Autodesk Inventor part; units mm, degrees
ref_plane "YZ Plane" through (0, 0, 0) normal (1, 0, 0) x (0, 1, 0)
ref_plane "XZ Plane" through (0, 0, 0) normal (0, 1, 0) x (-1, 0, 0)
ref_plane "XY Plane" through (0, 0, 0) normal (0, 0, 1) x (1, 0, 0)
sketch "스케치1" plane through (0, 0, 0) normal (0, 1, 0) x (-1, 0, 0)
  circle A0 centre (-0.1334, 0.1917) radius 4
  circle A1 centre (-0.1334, 0.1917) radius 11
  circle A2 centre (-0.1334, 0.1917) radius 11
  circle A3 centre (-0.1334, 0.1917) radius 8
  circle A4 centre (-0.1334, 8.1917) radius 1
  circle A5 centre (-5.7903, 5.8486) radius 1
  circle A6 centre (-8.1334, 0.1917) radius 1
  circle A7 centre (-5.7903, -5.4651) radius 1
  circle A8 centre (-0.1334, -7.8083) radius 1
  circle A9 centre (5.5235, -5.4651) radius 1
  circle A10 centre (7.8666, 0.1917) radius 1
  circle A11 centre (5.5235, 5.8486) radius 1
  line L0 (0, 0) -> (0, -10.8075)
  line L1 (10.8649, 0) -> (125.8649, 0)
  line L2 (125.8649, 0) -> (125.8649, -5)
  line L3 (125.8649, -5) -> (9.5643, -5)
  line L4 (125.8649, 0) -> (125.8649, 5)
  line L5 (125.8649, 5) -> (9.7601, 5)
  point P0 (9.5643, -5)
  point P1 (9.7601, 5)
  dimension "d2" = 16
  dimension "d3" = 2
  dimension "d4" = 360
  dimension "d5" = 115
  dimension "d6" = 5
  dimension "d7" = 5
extrude "돌출1" add sketch "스케치1" along normal blind 3 contours A1 | A1 L5 L4 L1 | L1 L2 L3 A1 | A10 A3 A9 A8 A7 A6 A5 A4 A11
fillet "모깎기1" radius 1 4 edges at (-9.7601, 1.5, 5) (-9.5643, 1.5, -5) (4.1334, 3, 0.1917) (11.1313, 3, 0.407)
sketch "스케치3" plane through (0, 0, 0) normal (0, -1, 0) x (1, 0, 0)
  arc A0 (-10.3673, 5) -> (-9.4922, 5.516) centre (-10.3673, 6) ccw
  arc A1 (-9.2892, -5.484) -> (-9.4922, 5.516) centre (0.1334, 0.1917) ccw
  arc A2 (-9.4922, 5.516) -> (-9.2892, -5.484) centre (0.1334, 0.1917) ccw
  arc A3 (-10.3673, 5) -> (-9.4922, 5.516) centre (-10.3673, 6) ccw
  arc A4 (-9.2892, -5.484) -> (-10.1458, -5) centre (-10.1458, -6) ccw
  arc A5 (-9.2892, -5.484) -> (-10.1458, -5) centre (-10.1458, -6) ccw
  line L0 (-125.8649, -5) -> (-125.8649, 5)
  line L1 (-10.1458, -5) -> (-125.8649, -5)
  line L2 (-125.8649, -5) -> (-125.8649, 5)
  line L3 (-125.8649, 5) -> (-10.3673, 5)
  point P0 (0, 0)
extrude "돌출3" add sketch "스케치3" along normal blind 2 contours A0 A2 A4 L1 L0 L3
thicken "두껍게 하기1" operation add thickness 3 both sides no extend neighbours no toward (0, -1, 0) faces at (3.6327, 0, 8.2973)
sketch "스케치4" plane through (-125.8649, 3, -5) normal (-1, 0, 0) x (0, 0, 1)
  circle A0 centre (5, -3) radius 1.5
  dimension "d20" = 3
extrude "돌출4" cut sketch "스케치4" against normal blind 4
properties part number "팔" material "ABS 플라스틱"
Can you work these out from the model? Positions are in its coordinate system, mm. A direction names the side the tool comes from. Give positions to 0.01 mm unless a question says otherwise; leave off trailing zeros. Loops run counter-clockwise (first coordinate to the right, second up) from the corner with the lowest first, then second, coordinate; pieces in that order, holes last. Notation, with made-up numbers: M 23.5,21 L 78.5,21 A21 cw 78.5,37 Z; hole C 33.25,-17.5 d10. An arc over 180 degrees is marked long. Answer in a Markdown table with one row per item.
1. If I drill on line 1 along X through (y, z) = (-1.25, -4.75); line 2 along X through (y, z) = (-0.25, 0.5); line 3 along X through (y, z) = (-0.75, -0.5), over which ranges is the centre line in solid material (lowest first)?
Taken from the geometry:
| item | result |
|---|---|
| line 1 | x = -125.86 to -6.22, -4.82 to 5.09, 6.49 to 9.96 |
| line 2 | x = -121.86 to -8.82, -6.92 to -3.85, 4.12 to 7.18, 9.08 to 11.13 |
| line 3 | x = -121.86 to -8.59, -7.14 to -3.81, 4.07 to 7.41, 8.86 to 11.11 |
2. Which directions (+Z, -Z, +X, -X, +Y, -Y) give clear straight access to the entire face, cutting with the end or side of a thin tool? Please do faces 1 (the flat face through (-57, 3, 0)), 2 (the flat face through (0, -3, -5)), 3 (the flat face through (-69, 0, -5)), 4 (the flat face through (-69, 0, 5)), 5 (the cylindrical face through (-123.89, 0.07, -1.5)).
Taken from the geometry:
| item | result |
|---|---|
| face 1 | +Z, -Z, +X, -X, +Y |
| face 2 | +Z, -Z, +X, -X, -Y |
| face 3 | -Z, -X, +Y, -Y |
| face 4 | +Z, -X, +Y, -Y |
| face 5 | -X |
3. Suppose I cut it at A-A on x = -73.5. Write out the boundary of the cut face in (y, z).
Taken from the geometry:
| item | result |
|---|---|
| outline | M -2,-5 L 3,-5 L 3,5 L -2,5 Z |
4. For pin 1 Ø1 at (x, y) = (-74.5, 2) entering from -Z; pin 2 Ø1 at (x, y) = (-96, -2) entering from +Z; pin 3 Ø12 at (x, z) = (-50.5, -1.5) entering from -Y, each with a flat end and sliding along its axis, tell me the tip position at first contact or that it passes through.
Taken from the geometry:
| item | result |
|---|---|
| pin 1 | stops at z = -5 |
| pin 2 | stops at z = 5 |
| pin 3 | stops at y = -2 |
5. Thinking about a two-plate mould opening in X: for faces 6 (the cylindrical face through (1.001, -0.465, -3.713)), 7 (the flat face through (-125.865, 2, 0)), 8 (the flat face through (-68, -2, 0)), which applies, released by +X, released by -X, zero draft, split by the parting line, or undercut?
Taken from the geometry:
| item | result |
|---|---|
| face 6 | undercut |
| face 7 | released by -X |
| face 8 | zero draft |
